Check sheet for the modelled part. Datum: model origin and axes. Units: mm. Face numbers are marked on the shaded views. A direction names the side the tool comes from. Coordinates: 2 decimals unless noted, no trailing zeros. Loops run counter-clockwise (first coordinate to the right, second up) from the corner with the lowest first, then second, coordinate; pieces in that order, holes last. Notation, with made-up numbers: (5, 37.5) - (37, 37.5) arc R14 cw to (37, 45.5) - close; hole circle Ø11 at (-34.5, -6.5). An arc over 180 degrees is marked (long way). Write each question's results on one line, items separated by ' | '. Start each with the question number.
1. Cross-section at C-C (y = 9.5). Record the cut outline in (x, z).
2. Thickness scan on line 1 (X direction, y = 1.3, z = -10.65); line 2 (Z direction, x = 0.5, y = 1.35); line 3 (Y direction, x = 8.25, z = -7.25). Record the ranges inside material, lowest first. Write a range as [from, to].
3. Cross-section at B-B (x = 0.5). Record the cut outline in (y, z), and give its area (4 significant figures).
4. Tool access check on the marked faces 1 and 2. Record the directions out of +Z, -Z, +X, -X, +Y, -Y that give a thin tool (end or side, any length) a straight path to the whole face; none if there is none.
5. Draft check along Z on the marked faces 3, 4 and 5. Enter one of: released by +Z, released by -Z, zero draft, split by the parting line, or undercut.
6. Gauge pin test, flat ends, axial feed: P1, Ø1.2, axis at y = 0.5, z = 1, coming from the +X side; P2, Ø2, axis at x = 10, z = -13.5, coming from the +Y side; P3, Ø1.6, axis at x = 10.5, z = -17, coming from the +Y side; P4, Ø1.6, axis at y = 1, z = -2, coming from the -X side. Record the tip position at first contact, or that the pin passes through.
7. Cross-section at D-D (z = -6.75). Record the cut outline in (x, y).
8. Cross-section at A-A (z = -10.65). Record the cut outline in (x, y), and give its area (3 significant figures).
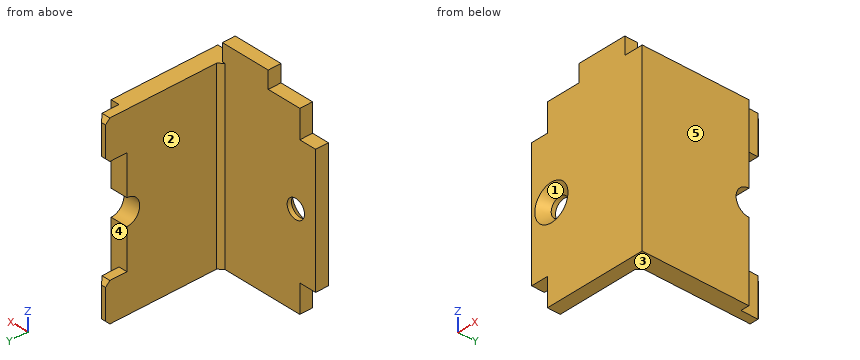
```python
from build123d import *

# Parameters (mm, degrees)
SKETCH1_W           = 12
SKETCH1_H           = 21.3
BOSS_EXTRUDE1_DEPTH = 1.5
SKETCH2_W           = 2
SKETCH2_H           = 21.3
BOSS_EXTRUDE2_DEPTH = 11
SKETCH3_W           = 2
SKETCH3_H           = 14.8
BOSS_EXTRUDE3_DEPTH = 1.5
SKETCH4_R           = 1.5
CUT_EXTRUDE1_DEPTH  = 2
CHAMFER1_SIZE       = 0.5
CUT_EXTRUDE2_REACH  = 3.5
SKETCH5_R           = 1.1
CHAMFER2_SIZE       = 1
SKETCH6_W           = 1
SKETCH6_H           = 4.5
BOSS_EXTRUDE4_DEPTH = 2.5
CHAMFER3_SIZE       = 0.5
SKETCH7_W           = 5.8
SKETCH7_H           = 1.5
BOSS_EXTRUDE5_DEPTH = 2


with BuildPart() as part:
    # Sketch1 → Boss-Extrude1 (new body)
    with BuildSketch(Plane(origin=(0, 0, 0), x_dir=(1, 0, 0), z_dir=(0, 1, 0))):
        with Locations((6, 10.65)):
            Rectangle(SKETCH1_W, SKETCH1_H)
    extrude(amount=BOSS_EXTRUDE1_DEPTH)

    # Sketch2 → Boss-Extrude2 (add)
    with BuildSketch(Plane(origin=(0, 1.5, 0), x_dir=(1, 0, 0), z_dir=(0, 1, 0))):
        with Locations((11, 10.65)):
            Rectangle(SKETCH2_W, SKETCH2_H)
    extrude(amount=BOSS_EXTRUDE2_DEPTH)

    # Sketch3 → Boss-Extrude3 (add)
    with BuildSketch(Plane(origin=(0, 1.5, 0), x_dir=(1, 0, 0), z_dir=(0, 1, 0))):
        with Locations((-1, 10.65)):
            Rectangle(SKETCH3_W, SKETCH3_H)
    extrude(amount=-BOSS_EXTRUDE3_DEPTH)

    # Sketch4 → Cut-Extrude1 (cut)
    with BuildSketch(Plane.ZY.offset(-10)):
        with Locations((-10.65, 12.5)):
            Circle(SKETCH4_R)
    extrude(amount=-CUT_EXTRUDE1_DEPTH, mode=Mode.SUBTRACT)

    # Chamfer1
    chamfer1_edges = [part.edges().sort_by_distance(p)[0] for p in [
        (10, 1.5, -10.65),
    ]]
    chamfer(chamfer1_edges, length=CHAMFER1_SIZE)

    # Sketch5 → Cut-Extrude2 (cut, up to next)
    with BuildSketch(Plane(origin=(0, 1.5, 0), x_dir=(1, 0, 0), z_dir=(0, 1, 0)), mode=Mode.PRIVATE) as cut_extrude2_sk1:
        with Locations((0.5, 10.65)):
            Circle(SKETCH5_R)
    cut_extrude2_tool1 = extrude(cut_extrude2_sk1.sketch, amount=-CUT_EXTRUDE2_REACH, mode=Mode.PRIVATE) & part.part
    add(cut_extrude2_tool1.solids().sort_by_distance((0.5, 1.5, -10.65))[0], mode=Mode.SUBTRACT)

    # Chamfer2
    chamfer2_edges = [part.edges().sort_by_distance(p)[0] for p in [
        (-0.6, 0, -10.65),
    ]]
    chamfer(chamfer2_edges, length=CHAMFER2_SIZE)

    # Sketch6 → Boss-Extrude4 (add)
    with BuildSketch(Plane(origin=(0, 12.5, 0), x_dir=(1, 0, 0), z_dir=(0, 1, 0))):
        with Locations((10.5, 2.25)):
            Rectangle(SKETCH6_W, SKETCH6_H)
        with Locations((10.5, 19.05)):
            Rectangle(SKETCH6_W, SKETCH6_H)
    extrude(amount=BOSS_EXTRUDE4_DEPTH)

    # Chamfer3
    chamfer3_edges = [part.edges().sort_by_distance(p)[0] for p in [
        (10.5, 15, -21.3),
        (11, 15, -19.05),
        (10.5, 15, -16.8),
        (10.5, 15, -4.5),
        (11, 15, -2.25),
        (10.5, 15, 0),
    ]]
    chamfer(chamfer3_edges, length=CHAMFER3_SIZE)

    # Sketch7 → Boss-Extrude5 (add)
    with BuildSketch(Plane.XY):
        with Locations((6.9, 0.75)):
            Rectangle(SKETCH7_W, SKETCH7_H)
    extrude(amount=BOSS_EXTRUDE5_DEPTH)


solid = part.part
```
Established:
1) outline: (10, -21.3) - (12, -21.3) - (12, 0) - (10, 0) - close
2) line 1: [-2, -0.6], [1.6, 12] | line 2: [-21.3, -11.75], [-9.55, 0] | line 3: [0, 1.5]
3) outline: (0, -21.3) - (1.5, -21.3) - (1.5, -11.75) - (1, -11.75) - (0, -12.75) - close; (0, -8.55) - (1, -9.55) - (1.5, -9.55) - (1.5, 0) - (0, 0) - close | area: 27.65 mm^2
4) face 1: -Y | face 2: +Z, -Z, -X, +Y
5) face 3: released by -Z | face 4: undercut | face 5: zero draft
6) P1: x = 9.8 | P2: y = 12.5 | P3: y = 15 | P4: x = 0
7) outline: (-2, 0) - (12, 0) - (12, 12.5) - (10, 12.5) - (10, 2) - (9.5, 1.5) - (-2, 1.5) - close
8) outline: (-2, 0) - (-1.6, 0) - (-0.6, 1) - (-0.6, 1.5) - (-2, 1.5) - close; (1.6, 1) - (2.6, 0) - (12, 0) - (12, 11) - (10, 11) - (10, 2) - (9.5, 1.5) - (1.6, 1.5) - close | area: 35.8 mm^2
